Geometry check sheet. Reference: the model listing, model coordinates, mm. A direction names the side the tool comes from. Round coordinates to 2 decimals unless told otherwise and drop trailing zeros. Write each loop counter-clockwise with the first axis right and the second up, starting at its lowest first coordinate (ties: lowest second). Pieces come first, ordered by that corner, then holes. Notation, with made-up numbers: (-24, -14.5) - (-4, -14.5) arc R30 ccw to (-4, 10.5) - close; hole circle Ø2 at (65, 39.25). An arc over 180 degrees is marked (long way). Return JSON: item names as keys, results as strings.
```python
from build123d import *

# Parameters (mm, degrees)
SKETCH1_W           = 113
SKETCH1_H           = 150
BOSS_EXTRUDE1_DEPTH = 3.1
SKETCH9_R           = 1.55
CUT_EXTRUDE7_DEPTH  = 94.9513704
SKETCH10_R          = 1.25
CUT_EXTRUDE8_DEPTH  = 94.9513704
SKETCH12_R          = 1.5
CUT_EXTRUDE9_DEPTH  = 94.9513704
SKETCH13_R          = 1.5
CUT_EXTRUDE10_DEPTH = 94.9513704
SKETCH14_W          = 15
SKETCH14_H          = 30
CUT_EXTRUDE11_DEPTH = 94.9513704
SKETCH16_R          = 1.375
CUT_EXTRUDE12_DEPTH = 94.9513704
SKETCH18_R          = 1.5
CUT_EXTRUDE13_DEPTH = 94.9513704
FILLET1_R           = 2
FILLET2_R           = 2.5


with BuildPart() as part:
    # Sketch1 → Boss-Extrude1 (new body)
    with BuildSketch(Plane.XY):
        Rectangle(SKETCH1_W, SKETCH1_H)
    extrude(amount=BOSS_EXTRUDE1_DEPTH)

    # Sketch9 → Cut-Extrude7 (cut, through all)
    with BuildSketch(Plane.XY.offset(3.1)):
        with Locations((-53.5, 72)):
            Circle(SKETCH9_R)
        with Locations((53.5, 72)):
            Circle(SKETCH9_R)
        with Locations((53.5, -72)):
            Circle(SKETCH9_R)
        with Locations((-53.5, -72)):
            Circle(SKETCH9_R)
    extrude(amount=-CUT_EXTRUDE7_DEPTH, mode=Mode.SUBTRACT)

    # Sketch10 → Cut-Extrude8 (cut, through all)
    with BuildSketch(Plane.XY.offset(3.1)):
        with BuildLine():
            ThreePointArc((37.5, 21.75), (36.616116524, 21.383883476), (36.25, 20.5))
            Line((36.25, 20.5), (37.5, 20.5))
            Line((37.5, 20.5), (37.5, 21.75))
        make_face()
        with BuildLine():
            Line((37.5, 20.5), (36.25, 20.5))
            ThreePointArc((36.25, 20.5), (37.5, 19.25), (38.75, 20.5))
            ThreePointArc((38.75, 20.5), (38.383883476, 21.383883476), (37.5, 21.75))
            Line((37.5, 21.75), (37.5, 20.5))
        make_face()
        with Locations((-20.5, 69.5)):
            Circle(SKETCH10_R)
        with Locations((37.5, 69.5)):
            Circle(SKETCH10_R)
        with Locations((-20.5, 20.5)):
            Circle(SKETCH10_R)
    extrude(amount=-CUT_EXTRUDE8_DEPTH, mode=Mode.SUBTRACT)

    # Sketch12 → Cut-Extrude9 (cut, through all)
    with BuildSketch(Plane.XY.offset(3.1)):
        with Locations((-38.25, -30.75)):
            Circle(SKETCH12_R)
        with Locations((-38.25, -69.25)):
            Circle(SKETCH12_R)
        with Locations((38.25, -69.25)):
            Circle(SKETCH12_R)
        with Locations((38.25, -30.75)):
            Circle(SKETCH12_R)
    extrude(amount=-CUT_EXTRUDE9_DEPTH, mode=Mode.SUBTRACT)

    # Sketch13 → Cut-Extrude10 (cut, through all)
    with BuildSketch(Plane.XY.offset(3.1)):
        with Locations((-7.5, -10)):
            Circle(SKETCH13_R)
        with Locations((7.5, -10)):
            Circle(SKETCH13_R)
    extrude(amount=-CUT_EXTRUDE10_DEPTH, mode=Mode.SUBTRACT)

    # Sketch14 → Cut-Extrude11 (cut, through all)
    with BuildSketch(Plane.XY.offset(3.1)):
        with Locations((42.5, -5)):
            Rectangle(SKETCH14_W, SKETCH14_H)
        with Locations((-42.5, -5)):
            Rectangle(SKETCH14_W, SKETCH14_H)
    extrude(amount=-CUT_EXTRUDE11_DEPTH, mode=Mode.SUBTRACT)

    # Sketch16 → Cut-Extrude12 (cut, through all)
    with BuildSketch(Plane(origin=(0, 0, 0), x_dir=(-1, 0, 0), z_dir=(0, 0, -1))):
        with Locations((-30.09, 26.71)):
            Circle(SKETCH16_R)
        with Locations((13.09, 26.71)):
            Circle(SKETCH16_R)
        with Locations((13.09, 63.29)):
            Circle(SKETCH16_R)
        with Locations((-30.09, 63.29)):
            Circle(SKETCH16_R)
    extrude(amount=-CUT_EXTRUDE12_DEPTH, mode=Mode.SUBTRACT)

    # Sketch18 → Cut-Extrude13 (cut, through all)
    with BuildSketch(Plane.XY.offset(3.1)):
        with Locations((-50, 28)):
            Circle(SKETCH18_R)
        with Locations((50, 28)):
            Circle(SKETCH18_R)
    extrude(amount=-CUT_EXTRUDE13_DEPTH, mode=Mode.SUBTRACT)

    # Fillet1
    fillet1_edges = [part.edges().sort_by_distance(p)[0] for p in [
        (-56.5, 75, 1.55),
        (56.5, 75, 1.55),
        (56.5, -75, 1.55),
        (-56.5, -75, 1.55),
    ]]
    fillet(fillet1_edges, radius=FILLET1_R)

    # Fillet2
    fillet2_edges = [part.edges().sort_by_distance(p)[0] for p in [
        (-50, 10, 1.55),
        (-35, 10, 1.55),
        (-35, -20, 1.55),
        (-50, -20, 1.55),
        (50, 10, 1.55),
        (50, -20, 1.55),
        (35, -20, 1.55),
        (35, 10, 1.55),
    ]]
    fillet(fillet2_edges, radius=FILLET2_R)


solid = part.part
```
(1) Section check C-C, the plane z = 1. Give the number of separate pieces and of enclosed holes in the cut face, plus the area to 3 significant figures.
Response values:
{"separate pieces": "1", "enclosed holes": "22", "area": "15,900 mm^2"}
(2) Gauge pin test, flat end, axial feed: pin 1 (3 mm diameter, centred on x = 30.09, y = 26.71, fed in from -Z). Record the tip position at first contact, or that the pin passes through.
Response values:
{"pin 1": "stops at z = 0"}
(3) Section check A-A, the plane y = -4.5. Enter the section's corners in (x, z), plus the area to 3 significant figures.
Response values:
{"outline": "(-56.5, 0) - (-50, 0) - (-50, 3.1) - (-56.5, 3.1) - close; (-35, 0) - (35, 0) - (35, 3.1) - (-35, 3.1) - close; (50, 0) - (56.5, 0) - (56.5, 3.1) - (50, 3.1) - close", "area": "257 mm^2"}
(4) Material ranges on line 1 along Y through (x, z) = (30.09, 1.5) (3 decimals); line 2 along Y through (x, z) = (-20.5, 2.15); line 3 along Y through (x, z) = (-38.25, 1.45), recorded low to high. Write a range as [from, to].
Response values:
{"line 1": "y = [-75, 25.335], [28.085, 61.915], [64.665, 75]", "line 2": "y = [-75, 19.25], [21.75, 68.25], [70.75, 75]", "line 3": "y = [-75, -70.75], [-67.75, -32.25], [-29.25, -20], [10, 75]"}
(5) Access from +Z, -Z, +X, -X, +Y, -Y to the whole of each face (thin tool, end or side, straight path). Record for faces 4 (the face through (56.5, -1, 2)), 5 (the face through (35, -5, 2)).
Response values:
{"face 4": "+Z, -Z, +X, +Y, -Y", "face 5": "+Z, -Z"}
(6) Section check B-B, the plane x = -42. Enter the section's corners in (y, z).
Response values:
{"outline": "(-75, 0) - (-20, 0) - (-20, 3.1) - (-75, 3.1) - close; (10, 0) - (75, 0) - (75, 3.1) - (10, 3.1) - close"}
(7) Release check for a two-part mould opening along Y. For faces 1 (the face through (-56.5, -1, 2)), 2 (the face through (-50, -5, 2)), 3 (the face through (-1, -75, 2)) record: pulls with the +Y half, pulls with the -Y half, needs draft (parallel to the pull), parting line crosses it, or undercut.
Response values:
{"face 1": "needs draft", "face 2": "undercut", "face 3": "pulls with the -Y half"}
